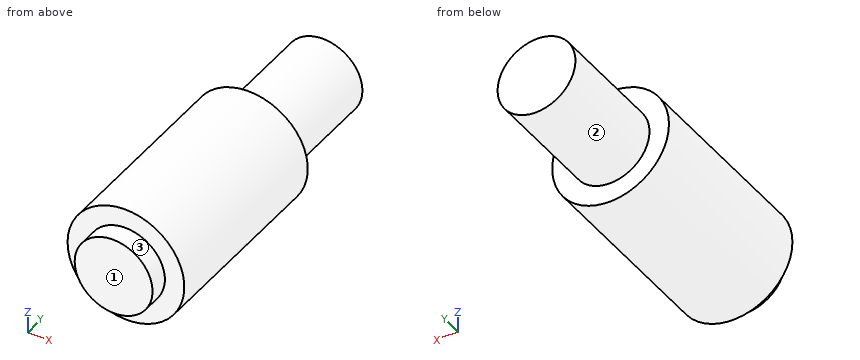
Autodesk Inventor part; units mm, degrees
ref_plane "YZ Plane" through (0, 0, 0) normal (1, 0, 0) x (0, 1, 0)
ref_plane "XZ Plane" through (0, 0, 0) normal (0, 1, 0) x (-1, 0, 0)
ref_plane "XY Plane" through (0, 0, 0) normal (0, 0, 1) x (1, 0, 0)
sketch "Sketch2" plane through (0, 0, 0) normal (0, 1, 0) x (-1, 0, 0)
  circle A0 centre (0, 0) radius 4
  circle A1 centre (0, 0) radius 6
  dimension "d4" = 8
  dimension "d5" = 12
extrude "Extrusion2" add sketch "Sketch2" along normal blind 20 contours A0 | A1
extrude "Extrusion3" add sketch "Sketch2" against normal blind 2 contours A0
sketch "Sketch3" plane through (0, 20, 0) normal (0, 1, 0) x (1, 0, 0)
  circle A0 centre (0, 0) radius 4
extrude "Extrusion4" add sketch "Sketch3" along normal blind 12
properties part number "springStub"
Source: CAD feature listing. Evaluate the final solid. Frame: model axes, mm. Face numbers are marked on the shaded views. A direction names the side the tool comes from. Round coordinates to 2 decimals unless told otherwise and drop trailing zeros. Write each loop counter-clockwise with the first axis right and the second up, starting at its lowest first coordinate (ties: lowest second). Pieces come first, ordered by that corner, then holes. Notation, with made-up numbers: M 19.5,-36 L 76.5,-36 A22 cw 76.5,-22 Z; hole C 61.5,84 d11. An arc over 180 degrees is marked long. Use CSV: the item, a comma, the result in double quotes. Start each with the question number.
Q1. Cut plane B-B on z = 2.5. Output: boundary loops of the cut face in (x, y), plus the area to 3 significant figures.
Q2. Line query: line 1 (Y direction, x = 0.5, z = -5); line 2 (Z direction, x = 5.25, y = 10); line 3 (Z direction, x = 4.25, y = 19.5). Output: solid intervals per line, ascending. Write a range as from..to.
Q3. Access query for the marked faces 1, 2 and 3. Directions: +Z, -Z, +X, -X, +Y, -Y. A direction counts if a zero-diameter tool reaches every point of the face in a straight line with its end or side. Return the directions, or none.
Q4. Cut plane D-D on y = 11. Output: boundary loops of the cut face in (x, z), plus the area to 3 significant figures.
Q5. Cut plane A-A on x = 0. Output: boundary loops of the cut face in (y, z).
Q6. Cut plane C-C on y = 27.5. Output: boundary loops of the cut face in (x, z), plus the area to 3 significant figures.
Q7. First-contact query: P1, Ø2, axis at x = 3, y = 1.5, coming from the -Z side; P2, Ø2, axis at x = -4.5, y = 5, coming from the +Z side. Flat tips, straight axial feed; report the tip coordinate or a pass-through.
Results found:
1,outline,"M -5.45,0 L -3.12,0 L -3.12,-2 L 3.12,-2 L 3.12,0 L 5.45,0 L 5.45,20 L 3.12,20 L 3.12,32 L -3.12,32 L -3.12,20 L -5.45,20 Z"
1,area,"306 mm^2"
2,line 1,"0..20"
2,line 2,"-2.9..2.9"
2,line 3,"-4.24..4.24"
3,face 1,"+Z, -Z, +X, -X, -Y"
3,face 2,"+Y"
3,face 3,"-Y"
4,outline,"C 0,0 d12"
4,area,"113 mm^2"
5,outline,"M -2,-4 L 0,-4 L 0,-6 L 20,-6 L 20,-4 L 32,-4 L 32,4 L 20,4 L 20,6 L 0,6 L 0,4 L -2,4 Z"
6,outline,"C 0,0 d8"
6,area,"50.3 mm^2"
7,P1,"z = -5.66"
7,P2,"z = 4.87"
